Here's how the part is built. I have some questions about the finished solid (model axes, mm). Face numbers are marked on the shaded views. A direction names the side the tool comes from. Round coordinates to 2 decimals unless told otherwise and drop trailing zeros. Loops run counter-clockwise (first coordinate to the right, second up) from the corner with the lowest first, then second, coordinate; pieces in that order, holes last. Notation, with made-up numbers: M -38.75,-22.5 L -4.75,-22.5 A21 ccw -4.75,8.5 Z; hole C 18.5,46 d1. An arc over 180 degrees is marked long. Put each result on its own line as item: value. Start each with the question number.
```python
from build123d import *

# Parameters (mm, degrees)
SKETCH1_W           = 30
SKETCH1_H           = 25
BOSS_EXTRUDE1_DEPTH = 25
CUT_EXTRUDE1_DEPTH  = 10
SKETCH3_W           = 10
SKETCH3_H           = 5
CUT_EXTRUDE2_DEPTH  = 30
CUT_EXTRUDE3_DEPTH  = 30
CUT_EXTRUDE5_DEPTH  = 10
SKETCH7_W           = 10
SKETCH7_H           = 10
CUT_EXTRUDE6_DEPTH  = 5


with BuildPart() as part:
    # Sketch1 → Boss-Extrude1 (new body)
    with BuildSketch(Plane.XY):
        with Locations((15, 12.5)):
            Rectangle(SKETCH1_W, SKETCH1_H)
    extrude(amount=BOSS_EXTRUDE1_DEPTH)

    # Sketch2 → Cut-Extrude1 (cut)
    with BuildSketch(Plane(origin=(30, 0, 0), x_dir=(0, 0, -1), z_dir=(1, 0, 0))):
        Polygon((-25, 25), (-25, 15), (-15, 25), align=None)
        Polygon((-10, 25), (0, 25), (0, 15), align=None)
    extrude(amount=-CUT_EXTRUDE1_DEPTH, mode=Mode.SUBTRACT)

    # Sketch3 → Cut-Extrude2 (cut)
    with BuildSketch(Plane.XY.offset(25)):
        with Locations((15, 2.5)):
            Rectangle(SKETCH3_W, SKETCH3_H)
    extrude(amount=-CUT_EXTRUDE2_DEPTH, mode=Mode.SUBTRACT)

    # Sketch4 → Cut-Extrude3 (cut)
    with BuildSketch(Plane.XY.offset(25)):
        Polygon((0, 25), (20, 25), (20, 15), (10, 15), (10, 20), (0, 20), align=None)
    extrude(amount=-CUT_EXTRUDE3_DEPTH, mode=Mode.SUBTRACT)

    # Sketch6 → Cut-Extrude5 (cut)
    with BuildSketch(Plane.ZY):
        Polygon((25, 20), (10, 15), (10, 20), align=None)
        Polygon((25, 0), (10, 0), (25, 5), align=None)
    extrude(amount=-CUT_EXTRUDE5_DEPTH, mode=Mode.SUBTRACT)

    # Sketch7 → Cut-Extrude6 (cut)
    with BuildSketch(Plane(origin=(0, 20, 0), x_dir=(1, 0, 0), z_dir=(0, 1, 0))):
        with Locations((5, -5)):
            Rectangle(SKETCH7_W, SKETCH7_H)
    extrude(amount=-CUT_EXTRUDE6_DEPTH, mode=Mode.SUBTRACT)


solid = part.part
```
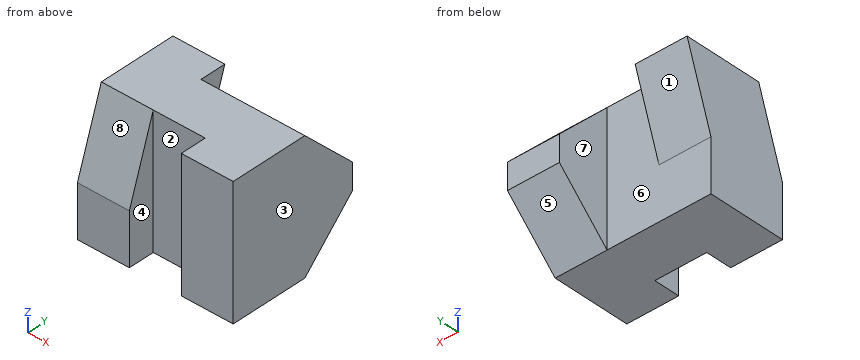
1) Suppose I cut it at C-C (x = 22). Write out the boundary of the cut face in (y, z), plus the area to 3 significant figures.
2) Suppose I cut it at B-B (z = 7.5). Write out the boundary of the cut face in (x, y), plus the area to 3 significant figures.
3) Suppose I cut it at D-D (z = 20.5). Write out the boundary of the cut face in (x, y).
4) I'm going to push flat-ended pins straight in: P1, Ø8, axis at x = 15, z = 15, coming from the -Y side; P2, Ø4, axis at x = 17, y = 16.5, coming from the -Z side; P3, Ø6, axis at x = 21, y = 22, coming from the +Z side; P4, Ø1, axis at x = 11.5, y = 17.5, coming from the +Z side. Where does each tip first touch, or does it pass through?
5) On a 3-axis mill with a long thin cutter (end or side, diameter ignored), from which of +Z, -Z, +X, -X, +Y, -Y can I reach the whole of each face in a straight line? I mean the marked faces 4, 5, 6, 7 and 8. Say none if no direction works.
6) If we mould it in two halves opening along X, with no side actions, what happens to the marked faces 1, 2 and 3? For each: pulls with the +X half, pulls with the -X half, needs draft (parallel to the pull), parting line crosses it, or undercut.
7) Suppose I cut it at A-A (y = 3.5). Write out the boundary of the cut face in (x, z).
8) If I drill on probe 1 along X at (y, z) = (16.5, 23.25); probe 2 along X at (y, z) = (21.25, 11.5); probe 3 along Y at (x, z) = (18.75, 15.25), over which ranges is the centre line in solid material (lowest first)? Write a range as from..to.
Results are:
1. outline: M 0,0 L 15,0 L 25,10 L 25,15 L 15,25 L 0,25 Z
1. area: 525 mm²
2. outline: M 0,0 L 10,0 L 10,5 L 20,5 L 20,0 L 30,0 L 30,22.5 L 20,22.5 L 20,15 L 0,15 Z
2. area: 475 mm²
3. outline: M 0,3.5 L 10,3.5 L 10,5 L 20,5 L 20,0 L 30,0 L 30,19.5 L 20,19.5 L 20,15 L 10,15 L 10,18.5 L 0,18.5 Z
4. P1: y = 5
4. P2: z = 0
4. P3: z = 21
4. P4: through
5. face 4: +Z, -Z, -Y
5. face 5: -Z, +X, -X, +Y
5. face 6: -Z, +Y
5. face 7: +Z, -Z, +Y
5. face 8: +Z, -X, -Y
6. face 1: needs draft
6. face 2: undercut
6. face 3: pulls with the +X half
7. outline: M 0,0 L 10,0 L 10,20.5 L 0,20.5 Z; M 20,0 L 30,0 L 30,25 L 20,25 Z
8. probe 1: 0..10, 20..30
8. probe 2: 20..30
8. probe 3: 5..15
